Can you work these out from the model? Positions are in its coordinate system, mm. Face numbers are marked on the shaded views. A direction names the side the tool comes from. Round coordinates to 2 decimals unless told otherwise and drop trailing zeros. Write each loop counter-clockwise with the first axis right and the second up, starting at its lowest first coordinate (ties: lowest second). Pieces come first, ordered by that corner, then holes. Notation, with made-up numbers: M 72,62.5 L 92,62.5 A14 ccw 92,79.5 Z; hole C 74,75 d6. An arc over 180 degrees is marked long. Answer as a JSON object with one key per item and string values. Group by question number.
1) Suppose I cut it at A-A, the plane z = -44. Write out the boundary of the cut face in (x, y).
2) Please list where these lines run through material, in increasing order: L1, parallel to X at y = 26.5, z = -0.5; L2, parallel to Z at x = 11, y = 32; L3, parallel to X at y = 16, z = -6.5. Write a range as [from, to].
3) On a 3-axis mill with a long thin cutter (end or side, diameter ignored), from which of +Z, -Z, +X, -X, +Y, -Y can I reach the whole of each face in a straight line? I mean the marked faces 1, 2 and 3. Say none if no direction works.
4) I'm going to push flat-ended pins straight in: pin 1 Ø11 at (y, z) = (27.5, -10.5) entering from -X; pin 2 Ø4 at (x, y) = (39, 27.5) entering from -Z; pin 3 Ø5.5 at (y, z) = (26.5, -44) entering from +X. Where does each tip first touch, or does it pass through?
5) Suppose I cut it at D-D, the plane x = -30.5. Write out the boundary of the cut face in (y, z), and give its area (3 significant figures).
6) Suppose I cut it at C-C, the plane y = 2. Write out the boundary of the cut face in (x, z).
7) Suppose I cut it at B-B, the plane x = 7.5. Write out the boundary of the cut face in (y, z), and give its area (3 significant figures).
from build123d import *

# Parameters (mm, degrees)
SKETCH_2_R          = 50
EXTRUDE_1_DEPTH     = 20
SKETCH_3_W          = 7
SKETCH_3_H          = 15
EXTRUDE_2_DEPTH     = 10
SKETCH_5_R          = 2.5
CUT_EXTRUDE_1_DEPTH = 111.157271919
SKETCH_7_W          = 22.619643184
SKETCH_7_H          = 7.983403476
SKETCH_7_W_2        = 20
SKETCH_7_H_2        = 5
EXTRUDE_3_DEPTH     = 15
SKETCH_8_W          = 22.619643184
SKETCH_8_H          = 7.983403476
CUT_EXTRUDE_2_DEPTH = 5
FILLET_1_R          = 2
FILLET_2_R          = 2


with BuildPart() as part:
    # 草图2 → 凸台-拉伸1 (new body)
    with BuildSketch(Plane(origin=(0, 0, 0), x_dir=(1, 0, 0), z_dir=(0, 1, 0))):
        with Locations(Location((5.130022326, 5.987717908, 0), (0, 0, 270))):
            Circle(SKETCH_2_R)
    extrude(amount=EXTRUDE_1_DEPTH)

    # 草图3 → 凸台-拉伸2 (add)
    with BuildSketch(Plane(origin=(0, 20, 0), x_dir=(1, 0, 0), z_dir=(0, 1, 0))):
        with Locations((-31.369977674, 7.5)):
            Rectangle(SKETCH_3_W, SKETCH_3_H)
        with Locations((41.630022326, 7.5)):
            Rectangle(SKETCH_3_W, SKETCH_3_H)
    extrude(amount=EXTRUDE_2_DEPTH)

    # 草图5 → 切除-拉伸1 (cut, through all)
    with BuildSketch(Plane.ZY.offset(34.869977674)):
        with Locations((-7.44529761, 25.652801918)):
            Circle(SKETCH_5_R)
    extrude(amount=-CUT_EXTRUDE_1_DEPTH, mode=Mode.SUBTRACT)

    # 草图7 → 凸台-拉伸3 (add)
    with BuildSketch(Plane(origin=(0, 20, 0), x_dir=(1, 0, 0), z_dir=(0, 1, 0))):
        with Locations((9.977088722, 44.289046493)):
            Rectangle(SKETCH_7_W, SKETCH_7_H)
        with Locations((10, 44.317993036)):
            Rectangle(SKETCH_7_W_2, SKETCH_7_H_2, mode=Mode.SUBTRACT)
    extrude(amount=EXTRUDE_3_DEPTH)

    # 草图8 → 切除-拉伸2 (cut)
    with BuildSketch(Plane.XZ):
        with Locations((9.977088722, -44.289046493)):
            Rectangle(SKETCH_8_W, SKETCH_8_H)
    extrude(amount=-CUT_EXTRUDE_2_DEPTH, mode=Mode.SUBTRACT)

    # 圆角1
    fillet_1_edges = [part.edges().sort_by_distance(p)[0] for p in [
        (-31.369977674, 30, -15),
    ]]
    fillet(fillet_1_edges, radius=FILLET_1_R)

    # 圆角2
    fillet_2_edges = [part.edges().sort_by_distance(p)[0] for p in [
        (41.630022326, 30, 0),
        (41.630022326, 30, -15),
        (-31.369977674, 30, 0),
    ]]
    fillet(fillet_2_edges, radius=FILLET_2_R)


solid = part.part
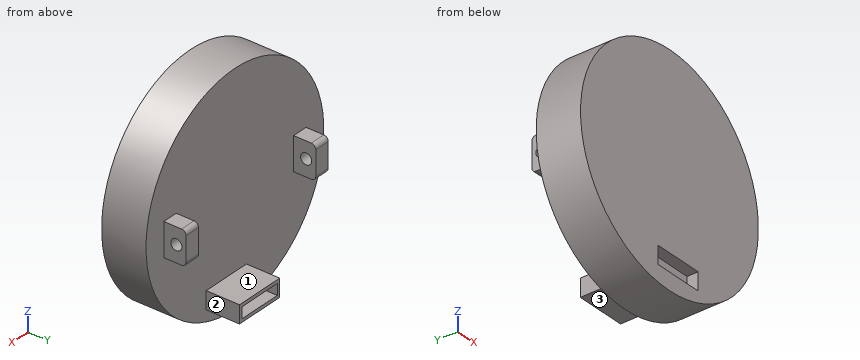
Results:
{
 "1": {"outline": "M -27.35,0 L -1.33,0 L -1.33,5 L 21.29,5 L 21.29,0 L 37.61,0 L 37.61,20 L 21.29,20 L 21.29,35 L 20,35 L 20,20 L 0,20 L 0,35 L -1.33,35 L -1.33,20 L -27.35,20 Z"},
 "2": {"L1": "[-34.87, -27.87], [38.13, 45.13]", "L2": "[-48.28, -46.82], [-41.82, -40.3]", "L3": "[-44.87, 55.13]"},
 "3": {"face 1": "+Z, +X, -X, +Y", "face 2": "+Z, -Z, +X, +Y", "face 3": "-Z, +X, -X, +Y"},
 "4": {"pin 1": "x = -34.87", "pin 2": "z = -15", "pin 3": "x = 21.29"},
 "5": {"outline": "M 0,-41.07 L 20,-41.07 L 20,-15 L 28,-15 A2 ccw 30,-13 L 30,-2 A2 ccw 28,0 L 20,0 L 20,29.09 L 0,29.09 Z; hole C 25.65,-7.45 d5", "area": "1,530 mm^2"},
 "6": {"outline": "C 5.13,-5.99 d100; hole M -1.33,-48.28 L 21.29,-48.28 L 21.29,-40.3 L -1.33,-40.3 Z"},
 "7": {"outline": "M 0,-55.93 L 20,-55.93 L 20,-48.28 L 35,-48.28 L 35,-46.82 L 20,-46.82 L 20,-41.82 L 35,-41.82 L 35,-40.3 L 20,-40.3 L 20,43.96 L 0,43.96 L 0,-40.3 L 5,-40.3 L 5,-48.28 L 0,-48.28 Z", "area": "2,000 mm^2"}
}
